The listing builds one solid part. Answer for the finished solid, in the listing's coordinates (mm). A direction names the side the tool comes from. Give positions to 0.01 mm unless a question says otherwise; leave off trailing zeros. Order: outer loops, then holes, each group sorted by start corner. A loop starts at its lowest first (then second) coordinate and runs counter-clockwise, first axis right, second up. Notation, with made-up numbers: (-30.5, -40) -> (-5.5, -40) arc R25 ccw to (-5.5, -16) -> close; hole circle Ø10 at (-14, 63). An arc over 180 degrees is marked (long way). Answer as a JSON object with one key per item and string values. Group by question number.
```python
from build123d import *

# Parameters (mm, degrees)
SKETCH1_W               = 13
SKETCH1_H               = 13
SKETCH1_W_2             = 11
SKETCH1_H_2             = 11
BOSS_EXTRUDE1_DEPTH     = 400
CUT_EXTRUDE1_DEPTH      = 1
CUT_EXTRUDE1_DEPTH_BACK = 14
CUT_EXTRUDE3_DEPTH      = 1
CUT_EXTRUDE3_DEPTH_BACK = 14


with BuildPart() as part:
    # Sketch1 → Boss-Extrude1 (new body)
    with BuildSketch(Plane(origin=(0, 0, 0), x_dir=(1, 0, 0), z_dir=(0, 1, 0))):
        Rectangle(SKETCH1_W, SKETCH1_H)
        Rectangle(SKETCH1_W_2, SKETCH1_H_2, mode=Mode.SUBTRACT)
    extrude(amount=BOSS_EXTRUDE1_DEPTH)

    # Sketch2 → Cut-Extrude1 (cut, two sides)
    with BuildSketch(Plane.ZY.offset(6.5)) as cut_extrude1_sk:
        Polygon((708.34637623, 805.211194246), (6.5, 400), (-6.5, 392.494446501), (-708.34637623, -12.716747746), (-1518.768764723, 1390.976004715), (-102.076012262, 2208.903946707), align=None)
    extrude(amount=CUT_EXTRUDE1_DEPTH, mode=Mode.SUBTRACT)
    extrude(cut_extrude1_sk.sketch, amount=-CUT_EXTRUDE1_DEPTH_BACK, mode=Mode.SUBTRACT)

    # Sketch3 → Cut-Extrude3 (cut, two sides)
    with BuildSketch(Plane.ZY.offset(6.5)) as cut_extrude3_sk:
        Polygon((708.34637623, -405.211194246), (6.5, 0), (-6.5, 7.505553499), (-708.34637623, 412.716747746), (-1518.768764723, -990.976004715), (-102.076012262, -1808.903946707), align=None)
    extrude(amount=CUT_EXTRUDE3_DEPTH, mode=Mode.SUBTRACT)
    extrude(cut_extrude3_sk.sketch, amount=-CUT_EXTRUDE3_DEPTH_BACK, mode=Mode.SUBTRACT)


solid = part.part
```
(1) For a pull along X with two mould halves and no side action, classify faces 3 (the flat face through (-5.5, 197, 0)), 4 (the flat face through (5.69, 396.3, 0.09)), 5 (the flat face through (-6.5, 197, 0)) as +X half, -X half, draft (parallel to the pull), parting line (faces both ways), or undercut.
(2) A cutting plane is placed at C-C (z = -1.25). Determine the outline of the cut face in (x, y), and give its area (3 significant figures).
(3) A cutting plane is placed at A-A (y = 92.5). Determine the outline of the cut face in (x, z).
(4) A cutting plane is placed at B-B (x = 3). Determine the outline of the cut face in (y, z).
(5) Which of the six approach directions +Z, -Z, +X, -X, +Y, -Y give full straight-line access (tool end or side, diameter ignored) to faces 1 (the flat face through (5.69, 3.7, 0.09)), 2 (the flat face through (5.5, 197, 0))?
(6) Find the intervals of material crossed by line 1 along Z through (x, y) = (2, 52.5), in increasing order. Write a range as [from, to].
Check sheet entries:
{
 "1": {"face 3": "undercut", "face 4": "draft", "face 5": "-X half"},
 "2": {"outline": "(-6.5, 4.47) -> (-5.5, 4.47) -> (-5.5, 395.53) -> (-6.5, 395.53) -> close; (5.5, 4.47) -> (6.5, 4.47) -> (6.5, 395.53) -> (5.5, 395.53) -> close", "area": "782 mm2"},
 "3": {"outline": "(-6.5, -6.5) -> (6.5, -6.5) -> (6.5, 6.5) -> (-6.5, 6.5) -> close; hole (-5.5, -5.5) -> (5.5, -5.5) -> (5.5, 5.5) -> (-5.5, 5.5) -> close"},
 "4": {"outline": "(0, 6.5) -> (0.58, 5.5) -> (399.42, 5.5) -> (400, 6.5) -> close; (6.93, -5.5) -> (7.51, -6.5) -> (392.49, -6.5) -> (393.07, -5.5) -> close"},
 "5": {"face 1": "-Z, +X, -X, -Y", "face 2": "+Y, -Y"},
 "6": {"line 1": "z = [-6.5, -5.5], [5.5, 6.5]"}
}
